```python
from build123d import *

# Parameters (mm, degrees)
SKETCH_1_W          = 32.7
SKETCH_1_H          = 29
SKETCH_1_R          = 1.5
EXTRUDE_1_DEPTH     = 10
CHAMFER_1_SIZE      = 3
CUT_EXTRUDE_1_DEPTH = 11
FILLET_1_R          = 1


with BuildPart() as part:
    # 草图1 → 凸台-拉伸1 (new body)
    with BuildSketch(Plane.XY):
        Rectangle(SKETCH_1_W, SKETCH_1_H)
        with Locations((-14.35, -10)):
            Circle(SKETCH_1_R, mode=Mode.SUBTRACT)
        with Locations((-14.35, 10)):
            Circle(SKETCH_1_R, mode=Mode.SUBTRACT)
        with Locations((14.35, 10)):
            Circle(SKETCH_1_R, mode=Mode.SUBTRACT)
        with Locations((14.35, -10)):
            Circle(SKETCH_1_R, mode=Mode.SUBTRACT)
        with Locations((-14.35, 0)):
            Circle(SKETCH_1_R, mode=Mode.SUBTRACT)
    extrude(amount=EXTRUDE_1_DEPTH)

    # 倒角1
    chamfer_1_edges = [part.edges().sort_by_distance(p)[0] for p in [
        (16.35, -14.5, 5),
        (-16.35, -14.5, 5),
        (-16.35, 14.5, 5),
        (16.35, 14.5, 5),
    ]]
    chamfer(chamfer_1_edges, length=CHAMFER_1_SIZE)

    # 草图2 → 切除-拉伸1 (cut, through all)
    with BuildSketch(Plane.XY.offset(10)):
        Polygon((-11, 7), (-8, 10), (8, 10), (11, 7), (11, -7), (8, -10), (-8, -10), (-11, -7), align=None)
    extrude(amount=-CUT_EXTRUDE_1_DEPTH, mode=Mode.SUBTRACT)

    # 圆角1
    fillet_1_edges = [part.edges().sort_by_distance(p)[0] for p in [
        (16.35, 11.5, 5),
        (16.35, -11.5, 5),
        (-13.35, -14.5, 5),
        (13.35, -14.5, 5),
        (-13.35, 14.5, 5),
        (13.35, 14.5, 5),
        (-16.35, 11.5, 5),
        (-16.35, -11.5, 5),
        (-8, 10, 5),
        (8, 10, 5),
        (11, 7, 5),
        (11, -7, 5),
        (8, -10, 5),
        (-8, -10, 5),
        (-11, -7, 5),
        (-11, 7, 5),
    ]]
    fillet(fillet_1_edges, radius=FILLET_1_R)


solid = part.part
```
The listing builds one solid part. Answer for the finished solid, in the listing's coordinates (mm). A direction names the side the tool comes from. Coordinates: 2 decimals unless noted, no trailing zeros. Loops run counter-clockwise (first coordinate to the right, second up) from the corner with the lowest first, then second, coordinate; pieces in that order, holes last. Notation, with made-up numbers: (22, 56.5) -> (55, 56.5) arc R14 cw to (55, 70.5) -> close; hole circle Ø8 at (32.25, -23). An arc over 180 degrees is marked (long way). Return JSON: item names as keys, results as strings. Group by question number.
(1) Given pin 1 Ø10 at (x, y) = (-12, 7.5) entering from -Z, flat-ended and moving along its own axis, determine where the tip first touches the part or whether it passes through.
(2) A cutting plane is placed at A-A on x = -6.5. Write down the section's boundary in (y, z), and give its area (3 significant figures).
(3) A cutting plane is placed at D-D on y = -3. Write down the section's boundary in (x, z).
(4) Find the intervals of material crossed by probe 1 along Y at (x, z) = (-7, 8); probe 2 along Y at (x, z) = (-14, 8.5); probe 3 along X at (y, z) = (-9.5, 3), in increasing order. Write a range as from..to.
(5) A cutting plane is placed at C-C on x = 14.35. Write down the section's boundary in (y, z).
(6) Which of the six approach directions +Z, -Z, +X, -X, +Y, -Y give full straight-line access (tool end or side, diameter ignored) to faces 5 (the flat face through (16.35, 0, 5)), 6 (the flat face through (-10, 8, 5))?
(7) A cutting plane is placed at B-B on y = 0. Write down the section's boundary in (x, z), and give its area (3 significant figures).
(8) Determine the mould class of faces 1 (the cylindrical face through (13.16, -10.91, 4.93)), 2 (the flat face through (0, -13, 0)), 3 (the flat face through (-11, 0, 5)), 4 (the flat face through (-14.83, 13.02, 4.93)) for opening direction Y: released by +Y, released by -Y, zero draft, split by the parting line, or undercut.
The answers:
{
 "1": {"pin 1": "stops at z = 0"},
 "2": {"outline": "(-14.5, 0) -> (-10, 0) -> (-10, 10) -> (-14.5, 10) -> close; (10, 0) -> (14.5, 0) -> (14.5, 10) -> (10, 10) -> close", "area": "90.0 mm^2"},
 "3": {"outline": "(-16.35, 0) -> (-11, 0) -> (-11, 10) -> (-16.35, 10) -> close; (11, 0) -> (16.35, 0) -> (16.35, 10) -> (11, 10) -> close"},
 "4": {"probe 1": "y = -14.5..-10, 10..14.5", "probe 2": "y = -13.85..-11.46, -8.54..-1.46, 1.46..8.54, 11.46..13.85", "probe 3": "x = -16.35..-15.76, -12.94..-8.5, 8.5..12.94, 15.76..16.35"},
 "5": {"outline": "(-13.5, 0) -> (-11.5, 0) -> (-11.5, 10) -> (-13.5, 10) -> close; (-8.5, 0) -> (8.5, 0) -> (8.5, 10) -> (-8.5, 10) -> close; (11.5, 0) -> (13.5, 0) -> (13.5, 10) -> (11.5, 10) -> close"},
 "6": {"face 5": "+Z, -Z, +X, +Y, -Y", "face 6": "+Z, -Z"},
 "7": {"outline": "(-16.35, 0) -> (-15.85, 0) -> (-15.85, 10) -> (-16.35, 10) -> close; (-12.85, 0) -> (-11, 0) -> (-11, 10) -> (-12.85, 10) -> close; (11, 0) -> (16.35, 0) -> (16.35, 10) -> (11, 10) -> close", "area": "77.0 mm^2"},
 "8": {"face 1": "undercut", "face 2": "zero draft", "face 3": "undercut", "face 4": "released by +Y"}
}
